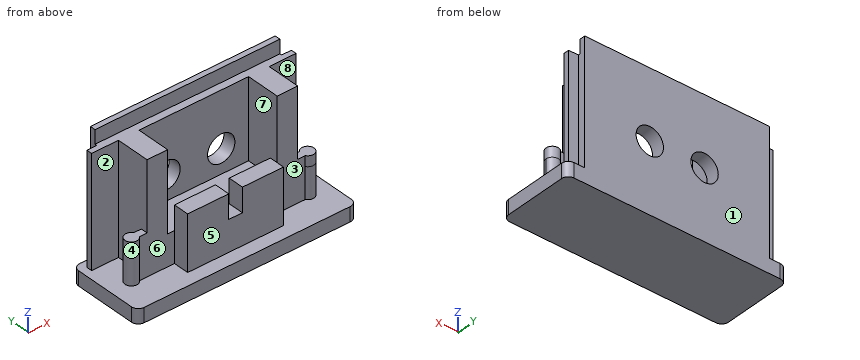
```python
from build123d import *

# Parameters (mm, degrees)
F1_DEPTH  = 2.1
F2_W      = 27
F2_H      = 1.1
F3_DEPTH  = 4.5
F4_DEPTH  = 11.5
F5_R      = 2
F6_DEPTH  = 25
F7_W      = 22
F7_H      = 3.925
F8_DEPTH  = 4.5
F10_DEPTH = 11.5
F11_W     = 6
F11_H     = 2.275
F12_DEPTH = 8
F13_W     = 27
F13_H     = 0.8
F14_DEPTH = 2
F15_W     = 2
F15_H     = 2.275
F16_DEPTH = 4.5
F18_DEPTH = 10


with BuildPart() as f1:
    # F0 (on Top) → F1 (new body)
    with BuildSketch(Plane.XY):
        with BuildLine():
            Line((15.05, 5.55), (-15.05, 5.55))
            ThreePointArc((-15.05, 5.55), (-15.7571067812, 5.2571067812), (-16.05, 4.55))
            Line((-16.05, 4.55), (-16.05, -4.55))
            ThreePointArc((-16.05, -4.55), (-15.7571067812, -5.2571067812), (-15.05, -5.55))
            Line((-15.05, -5.55), (15.05, -5.55))
            ThreePointArc((15.05, -5.55), (15.7571067812, -5.2571067812), (16.05, -4.55))
            Line((16.05, -4.55), (16.05, 4.55))
            ThreePointArc((16.05, 4.55), (15.7571067812, 5.2571067812), (15.05, 5.55))
        make_face()
    extrude(amount=F1_DEPTH)

    # F2 (on face) → F3 (join)
    with BuildSketch(Plane.XY.offset(2.1)):
        with BuildLine():
            ThreePointArc((13.8, -0.775), (13.1355497201, 0.1125465303), (12.0967808792, -0.275))
            Line((12.0967808792, -0.275), (12.875, -0.275))
            Line((12.875, -0.275), (12.875, -1.275))
            Line((12.875, -1.275), (12.0967808792, -1.275))
            ThreePointArc((12.0967808792, -1.275), (13.1355497201, -1.6625465303), (13.8, -0.775))
        make_face()
        with BuildLine():
            ThreePointArc((-12.0967808792, -0.275), (-11.9874534697, -0.5144502799), (-11.95, -0.775))
            ThreePointArc((-11.95, -0.775), (-11.9874534697, -1.0355497201), (-12.0967808792, -1.275))
            Line((-12.0967808792, -1.275), (12.0967808792, -1.275))
            ThreePointArc((12.0967808792, -1.275), (11.95, -0.775), (12.0967808792, -0.275))
            Line((12.0967808792, -0.275), (-12.0967808792, -0.275))
        make_face()
        with BuildLine():
            Line((12.875, -0.275), (12.0967808792, -0.275))
            ThreePointArc((12.0967808792, -0.275), (11.95, -0.775), (12.0967808792, -1.275))
            Line((12.0967808792, -1.275), (12.875, -1.275))
            Line((12.875, -1.275), (12.875, -0.275))
        make_face()
        with BuildLine():
            Line((-12.875, -0.275), (-12.0967808792, -0.275))
            ThreePointArc((-12.0967808792, -0.275), (-13.8, -0.775), (-12.0967808792, -1.275))
            Line((-12.0967808792, -1.275), (-12.875, -1.275))
            Line((-12.875, -1.275), (-12.875, -0.275))
        make_face()
        with BuildLine():
            ThreePointArc((-12.0967808792, -1.275), (-11.9874534697, -1.0355497201), (-11.95, -0.775))
            ThreePointArc((-11.95, -0.775), (-11.9874534697, -0.5144502799), (-12.0967808792, -0.275))
            Line((-12.0967808792, -0.275), (-12.875, -0.275))
            Line((-12.875, -0.275), (-12.875, -1.275))
            Line((-12.875, -1.275), (-12.0967808792, -1.275))
        make_face()
        Polygon((13.5, 4.45), (-13.5, 4.45), (-14.925, 4.45), (-14.925, 3.65), (14.925, 3.65), (14.925, 4.45), align=None)
        with Locations((0, 5)):
            Rectangle(F2_W, F2_H)
    extrude(amount=F3_DEPTH)

    # F4 (add): a face of the model
    f4_faces = [f1.faces().sort_by_distance(p)[0] for p in [
        (0, 4.5765957447, 6.6),
    ]]
    extrude(f4_faces, amount=F4_DEPTH)

    # F5 (on face) → F6 (cut)
    with BuildSketch(Plane(origin=(0, 5.55, 0), x_dir=(-1, 0, 0), z_dir=(0, 1, 0))):
        with Locations((4, 10.1)):
            Circle(F5_R)
        with Locations((-4, 10.1)):
            Circle(F5_R)
    extrude(amount=-F6_DEPTH, mode=Mode.SUBTRACT)

    # F7 (on face) → F8 (join, through all)
    with BuildSketch(Plane.XY.offset(2.1)):
        with Locations((0, 1.6875)):
            Rectangle(F7_W, F7_H)
    extrude(amount=F8_DEPTH)

    # F9 (on face) → F10 (join, through all)
    with BuildSketch(Plane.XY.offset(6.6)):
        with BuildLine():
            Line((-11, -0.275), (-12.0967808792, -0.275))
            ThreePointArc((-12.0967808792, -0.275), (-13.8, -0.775), (-12.0967808792, -1.275))
            Line((-12.0967808792, -1.275), (-8, -1.275))
            Line((-8, -1.275), (-8, 3.65))
            Line((-8, 3.65), (-11, 3.65))
            Line((-11, 3.65), (-11, -0.275))
        make_face()
        with BuildLine():
            Line((8, 3.65), (8, -1.275))
            Line((8, -1.275), (12.0967808792, -1.275))
            ThreePointArc((12.0967808792, -1.275), (13.8, -0.775), (12.0967808792, -0.275))
            Line((12.0967808792, -0.275), (11, -0.275))
            Line((11, -0.275), (11, 3.65))
            Line((11, 3.65), (8, 3.65))
        make_face()
    extrude(amount=F10_DEPTH)

    # F11 (on face) → F12 (join)
    with BuildSketch(Plane.XY.offset(2.1)):
        with Locations((-4, -2.4125)):
            Rectangle(F11_W, F11_H)
        with Locations((4, -2.4125)):
            Rectangle(F11_W, F11_H)
    extrude(amount=F12_DEPTH)

    # F13 (on face) → F14 (join)
    with BuildSketch(Plane.XY.offset(18.1)):
        with Locations((0, 5.15)):
            Rectangle(F13_W, F13_H)
    extrude(amount=F14_DEPTH)

    # F15 (on face) → F16 (join, through all)
    with BuildSketch(Plane.XY.offset(2.1)):
        with Locations((0, -2.4125)):
            Rectangle(F15_W, F15_H)
    extrude(amount=F16_DEPTH)

    # F17 (on face) → F18 (cut)
    with BuildSketch(Plane.XY.offset(18.1)):
        with BuildLine():
            Line((-11, -1.275), (-11, -0.275))
            Line((-11, -0.275), (-12.0967808792, -0.275))
            ThreePointArc((-12.0967808792, -0.275), (-13.8, -0.775), (-12.0967808792, -1.275))
            Line((-12.0967808792, -1.275), (-11, -1.275))
        make_face()
        with BuildLine():
            Line((12.0967808792, -0.275), (11, -0.275))
            Line((11, -0.275), (11, -1.275))
            Line((11, -1.275), (12.0967808792, -1.275))
            ThreePointArc((12.0967808792, -1.275), (13.8, -0.775), (12.0967808792, -0.275))
        make_face()
    extrude(amount=-F18_DEPTH, mode=Mode.SUBTRACT)


solid = f1.part
```
Could you check a few things on this model? Use its own coordinates, in mm. Face numbers are marked on the shaded views. A direction names the side the tool comes from. Round coordinates to 2 decimals unless told otherwise and drop trailing zeros. Loops run counter-clockwise (first coordinate to the right, second up) from the corner with the lowest first, then second, coordinate; pieces in that order, holes last.
Q1. I want a section at D-D (y = 1.75). Write out the boundary of the cut face in (x, z).
Q2. Thinking about a two-plate mould opening in Y: for the marked faces 6, 7 and 8, which applies, pulls with the +Y half, pulls with the -Y half, needs draft (parallel to the pull), parting line crosses it, or undercut?
Q3. I want a section at B-B (x = -7.5). Write out the boundary of the cut face in (y, z) (3 decimals), and give its area (3 significant figures).
Q4. On a 3-axis mill with a long thin cutter (end or side, diameter ignored), from which of +Z, -Z, +X, -X, +Y, -Y can I reach the whole of each face in a straight line? I mean the marked faces 1, 2, 3, 4 and 5. Say none if no direction works.
Q5. I want a section at C-C (z = 9.5). Give the number of separate pieces and of enclosed holes in the cut face, and give its area (3 significant figures).
Q6. I want a section at A-A (x = 4). Write out the boundary of the cut face in (y, z) (3 decimals), and give its area (3 significant figures).
Q7. Please list where these lines run through material, in increasing order: L1, parallel to Z at x = -4, y = 5.1; L2, parallel to Z at x = -4, y = 4.15; L3, parallel to Z at x = -4, y = 1.
Q8. For P1, Ø2.5, axis at y = -2.5, z = 6.5, coming from the +X side; P2, Ø1, axis at y = 2, z = 12.5, coming from the +X side; P3, Ø1.6, axis at x = -14.5, z = 8, coming from the +Y side; P4, Ø3, axis at y = -4, z = 16.5, coming from the -X side, each with a flat end and sliding along its axis, tell me the tip position at first contact or that it passes through.
Answer below:
1. outline: (-16.05, 0) - (16.05, 0) - (16.05, 2.1) - (11, 2.1) - (11, 18.1) - (8, 18.1) - (8, 6.6) - (-8, 6.6) - (-8, 18.1) - (-11, 18.1) - (-11, 2.1) - (-16.05, 2.1) - close
2. face 6: pulls with the -Y half
2. face 7: needs draft
2. face 8: undercut
3. outline: (-5.55, 0) - (5.55, 0) - (5.55, 20.1) - (4.75, 20.1) - (4.75, 18.1) - (3.65, 18.1) - (3.65, 6.6) - (-1.275, 6.6) - (-1.275, 2.1) - (-5.55, 2.1) - close
3. area: 77.5 mm2
4. face 1: +Z, -Z, +X, -X, +Y
4. face 2: +Z, -X
4. face 3: +Z, -Y
4. face 4: +Z
4. face 5: +Z, +X, -X, -Y
5. separate pieces: 5
5. enclosed holes: 0
5. area: 95.9 mm2
6. outline: (-5.55, 0) - (5.55, 0) - (5.55, 8.1) - (3.65, 8.1) - (3.65, 6.6) - (-1.275, 6.6) - (-1.275, 10.1) - (-3.55, 10.1) - (-3.55, 2.1) - (-5.55, 2.1) - close; (3.65, 12.1) - (5.55, 12.1) - (5.55, 20.1) - (4.75, 20.1) - (4.75, 18.1) - (3.65, 18.1) - close
6. area: 88.1 mm2
7. L1: z = 0 to 8.1, 12.1 to 20.1
7. L2: z = 0 to 8.1, 12.1 to 18.1
7. L3: z = 0 to 6.6
8. P1: stops at x = 13.67
8. P2: stops at x = 11
8. P3: stops at y = 4.45
8. P4: passes through
